```python
from build123d import *

# Parameters (mm, degrees)
SKETCH_1_R               = 23.5
SKETCH_1_R_2             = 21
EXTRUDE_1_DEPTH          = 15
SKETCH_2_R               = 1.25
CUT_EXTRUDE_1_DEPTH      = 27
PATTERN_CIRCULAR_1_COUNT = 4
SKETCH_3_R               = 22
EXTRUDE_2_DEPTH          = 2
SKETCH_4_R               = 1.25
CUT_EXTRUDE_2_DEPTH      = 2
SKETCH_5_R               = 16.5
EXTRUDE_4_DEPTH          = 10
SKETCH_6_R               = 4
CUT_EXTRUDE_5_DEPTH      = 10
SKETCH_8_R               = 1.25
CUT_EXTRUDE_6_DEPTH      = 43
PATTERN_CIRCULAR_2_COUNT = 4


with BuildPart() as part:
    # 草图1 → 凸台-拉伸1 (new body)
    with BuildSketch(Plane.XY):
        Circle(SKETCH_1_R)
        Circle(SKETCH_1_R_2, mode=Mode.SUBTRACT)
    extrude(amount=EXTRUDE_1_DEPTH)

    # 草图2 → 切除-拉伸1 (cut, symmetric)
    with BuildSketch(Plane(origin=(0, 0, 0), x_dir=(0, 0, -1), z_dir=(1, 0, 0))):
        with Locations((-5, 0)):
            Circle(SKETCH_2_R)
    cut_extrude_1 = extrude(amount=CUT_EXTRUDE_1_DEPTH, both=True, mode=Mode.SUBTRACT)

    # 阵列(圆周)1: 切除-拉伸1 ×4 about axis
    pattern_circular_1_axis = Axis((0, 0, 15), (0, 0, -1))
    for i in range(1, PATTERN_CIRCULAR_1_COUNT):
        add(cut_extrude_1.rotate(pattern_circular_1_axis, i * 360 / PATTERN_CIRCULAR_1_COUNT), mode=Mode.SUBTRACT)

    # 草图3 → 凸台-拉伸2 (add)
    with BuildSketch(Plane.XY.offset(15)):
        Circle(SKETCH_3_R)
    extrude(amount=EXTRUDE_2_DEPTH)

    # 草图4 → 切除-拉伸2 (cut)
    with BuildSketch(Plane.XY.offset(17)):
        with Locations((15.5, 0)):
            Circle(SKETCH_4_R)
        with Locations((0, -15.5)):
            Circle(SKETCH_4_R)
        with Locations((-15.5, 0)):
            Circle(SKETCH_4_R)
        with Locations((0, 15.5)):
            Circle(SKETCH_4_R)
    extrude(amount=-CUT_EXTRUDE_2_DEPTH, mode=Mode.SUBTRACT)

    # 草图5 → 凸台-拉伸4 (add)
    with BuildSketch(Plane.XY.offset(17)):
        with Locations(Location((0, 0, 0), (0, 0, 182.687298331))):
            Circle(SKETCH_5_R)
    extrude(amount=EXTRUDE_4_DEPTH)

    # 草图6 → 切除-拉伸5 (cut)
    with BuildSketch(Plane.XY.offset(27)):
        with Locations((0, -15.5)):
            Circle(SKETCH_6_R)
        with Locations((-15.5, 0)):
            Circle(SKETCH_6_R)
        with Locations((0, 15.5)):
            Circle(SKETCH_6_R)
        with Locations((15.5, 0)):
            Circle(SKETCH_6_R)
    extrude(amount=-CUT_EXTRUDE_5_DEPTH, mode=Mode.SUBTRACT)

    # 草图8 → 切除-拉伸6 (cut)
    with BuildSketch(Plane(origin=(11.66726189, 11.66726189, 0), x_dir=(0, 0, -1), z_dir=(0.7071067811865561, 0.7071067811865389, 0))):
        with Locations(Location((-22, 0, 0), (0, 0, 90))):
            Circle(SKETCH_8_R)
    cut_extrude_6 = extrude(amount=-CUT_EXTRUDE_6_DEPTH, mode=Mode.SUBTRACT)

    # 阵列(圆周)2: 切除-拉伸6 ×4 about axis
    pattern_circular_2_axis = Axis((0, 0, 27), (0, 0, 1))
    for i in range(1, PATTERN_CIRCULAR_2_COUNT):
        add(cut_extrude_6.rotate(pattern_circular_2_axis, i * 360 / PATTERN_CIRCULAR_2_COUNT), mode=Mode.SUBTRACT)


solid = part.part
```
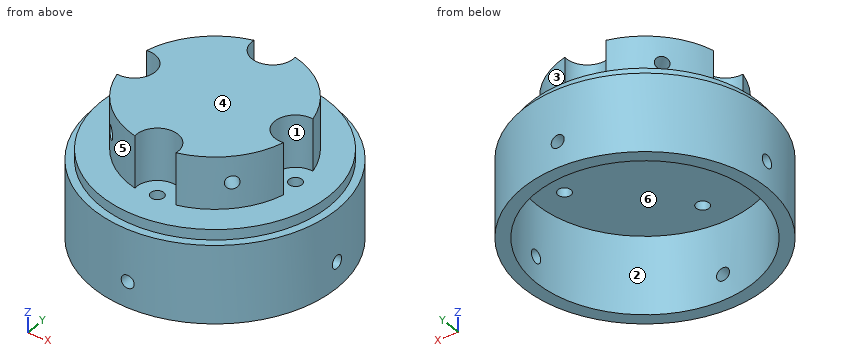
Verification items for the finished model (mm, model axes). Face numbers are marked on the shaded views. A direction names the side the tool comes from. Round coordinates to 2 decimals unless told otherwise and drop trailing zeros. Order: outer loops, then holes, each group sorted by start corner. A loop starts at its lowest first (then second) coordinate and runs counter-clockwise, first axis right, second up. Notation, with made-up numbers: (59.25, -37) - (78.25, -37) arc R23 ccw to (78.25, -18) - close; hole circle Ø2 at (-20.5, -37). An arc over 180 degrees is marked (long way). Use CSV: the item, a comma, the result in double quotes. Start each with the question number.
1) Section check A-A, the plane z = 5. Record the cut outline in (x, y).
2) Thickness scan on L1, parallel to Y at x = 0, z = 16.15; L2, parallel to Y at x = -1, z = 16.5; L3, parallel to Y at x = 0, z = 10.5. Record the ranges inside material, lowest first.
3) Access from +Z, -Z, +X, -X, +Y, -Y to the whole of each face (thin tool, end or side, straight path). Record for the marked faces 1, 2 and 3.
4) Section check B-B, the plane z = 14.25. Record the cut outline in (x, y), plus the area to 3 significant figures.
5) Go/stop test with flat-tipped pins: P1, Ø4, axis at x = 0, y = -15.5, coming from the -Z side; P2, Ø3, axis at x = -14, z = 18, coming from the -Y side; P3, Ø8, axis at y = -12, z = 13, coming from the -X side. Record where each tip stops, or that it passes through.
6) Section check C-C, the plane y = -7. State how many separate pieces and enclosed holes the cut face has, plus the area to 3 significant figures.
7) Mould release check, pull along Y, two halves, no side actions. Record for the marked faces 4, 5 and 6: +Y half, -Y half, draft (parallel to the pull), parting line (faces both ways), or undercut.
Answers:
1,outline,"(-23.47, -1.25) arc R23.5 ccw to (-1.25, -23.47) - (-1.25, -20.96) arc R21 cw to (-20.96, -1.25) - close; (-23.47, 1.25) - (-20.96, 1.25) arc R21 cw to (-1.25, 20.96) - (-1.25, 23.47) arc R23.5 ccw to start; (1.25, -23.47) arc R23.5 ccw to (23.47, -1.25) - (20.96, -1.25) arc R21 cw to (1.25, -20.96) - close; (1.25, 20.96) arc R21 cw to (20.96, 1.25) - (23.47, 1.25) arc R23.5 ccw to (1.25, 23.47) - close"
2,L1,"y = -22 to -16.75, -14.25 to 14.25, 16.75 to 22"
2,L2,"y = -21.98 to -16.25, -14.75 to 14.75, 16.25 to 21.98"
2,L3,"y = -23.5 to -21, 21 to 23.5"
3,face 1,"+Z"
3,face 2,"-Z"
3,face 3,"+Z, +X, +Y"
4,outline,"circle Ø47 at (0, 0); hole circle Ø42 at (0, 0)"
4,area,"350 mm²"
5,P1,"stops at z = 15"
5,P2,"stops at y = -17.83"
5,P3,"stops at x = -22.1"
6,separate pieces,"1"
6,enclosed holes,"2"
6,area,"447 mm²"
7,face 4,"draft"
7,face 5,"-Y half"
7,face 6,"undercut"
